The model under review builds one solid part; all positions refer to its coordinate system, in mm. A direction names the side the tool comes from. Round coordinates to 2 decimals unless told otherwise and drop trailing zeros. Order: outer loops, then holes, each group sorted by start corner. A loop starts at its lowest first (then second) coordinate and runs counter-clockwise, first axis right, second up.
1) Mouldability with a two-part tool opening along X and no side actions: class faces 4 (the face through (180.462, 10.81, -33.792)), 5 (the face through (239.15, -458.02, -15.02)), 6 (the face through (329.074, -455, -23)) as pulls with the +X half, pulls with the -X half, needs draft (parallel to the pull), parting line crosses it, or undercut.
2) Consider section A-A (z = 0). Give the boundary of the cut face in (x, y).
3) Consider section C-C (y = 411.5). Give the boundary of the cut face in (x, z).
4) Machinability: for faces 1 (the face through (-284, 306.407, -23)), 2 (the face through (-88.72, 495.28, -2.2)), 3 (the face through (-379.026, 381.199, -2.198)), which of the approach directions +Z, -Z, +X, -X, +Y, -Y give a long, thin tool a straight path to every point of the face, cutting with its end or side? Answer none if there is none.
5) To check wall thickness, follow L1, parallel to X at y = -121, z = 2.5; L2, parallel to X at y = -84.5, z = -23; L3, parallel to Y at x = 105, z = -45. State the ranges of each line that lie inside material, in increasing order.
6) Consider section B-B (x = 29.5). Give the boundary of the cut face in (y, z), then the cut area to 3 significant figures.
7) Clearance check with flat-ended pins moving along their axes: P1, Ø10, axis at x = -288.5, z = 9, coming from the +Y side; P2, Ø4, axis at y = -275, z = 21.5, coming from the +X side; P3, Ø2, axis at y = 147, z = 47.5, coming from the -X side. State where each tip first meets the part, or that it passes through.
8) Consider section D-D (y = -394.5). Give the boundary of the cut face in (x, z).
from build123d import *

# Parameters (mm, degrees)
SKETCH8_R   = 60
SKETCH8_R_2 = 50


with BuildPart() as part:
    # Sweep-Thin1: sweep along a path in Sketch1
    with BuildLine(Plane.XY) as sweep_thin1_path:
        Line((-329.073983606, 306.407118431), (-329.073983606, 445.327817433))
        Line((-329.073983606, 445.327817433), (143.609908522, 445.327817433))
        Line((143.609908522, 445.327817433), (143.609908522, -410.327817433))
        Line((143.609908522, -410.327817433), (329.073983606, -410.327817433))
    # Sketch8 → Sweep-Thin1 (sweep)
    with BuildSketch(Plane(origin=(0, 306.407118431, 0), x_dir=(1, 0, 0), z_dir=(0, 1, 0))):
        with Locations((-329.073983606, 0)):
            Circle(SKETCH8_R)
        with Locations((-329.073983606, 0)):
            Circle(SKETCH8_R_2, mode=Mode.SUBTRACT)
    sweep(path=sweep_thin1_path.line, transition=Transition.RIGHT)


solid = part.part
Answer below:
1. face 4: undercut
1. face 5: needs draft
1. face 6: pulls with the +X half
2. outline: (-389.07, 306.41) - (-379.07, 306.41) - (-379.07, 495.33) - (193.61, 495.33) - (193.61, -360.33) - (329.07, -360.33) - (329.07, -350.33) - (203.61, -350.33) - (203.61, 505.33) - (-389.07, 505.33) - close; (-279.07, 306.41) - (-269.07, 306.41) - (-269.07, 385.33) - (83.61, 385.33) - (83.61, -470.33) - (329.07, -470.33) - (329.07, -460.33) - (93.61, -460.33) - (93.61, 395.33) - (-279.07, 395.33) - close
3. outline: (-295.25, -49.55) - (109.78, -49.55) arc R60 ccw (long way) to (109.78, 49.55) - (-295.25, 49.55) arc R60 ccw (long way) to start; hole (-295.25, -36.82) - (109.78, -36.82) arc R50 ccw (long way) to (109.78, 36.82) - (-295.25, 36.82) arc R50 ccw (long way) to start
4. face 1: +Z, -Z, -X, -Y
4. face 2: none
4. face 3: -Y
5. L1: x = 83.66 to 93.67, 193.55 to 203.56
5. L2: x = 88.19 to 99.21, 188.01 to 199.03
5. L3: y = -450.01 to 423.53, 467.12 to 485.01
6. outline: circle Ø120 at (445.33, 0); hole circle Ø100 at (445.33, 0)
6. area: 3,460 mm2
7. P1: stops at y = 505.19
7. P2: stops at x = 200.35
7. P3: stops at x = 105.69
8. outline: (159.44, -57.87) - (329.07, -57.87) - (329.07, -47.43) - (159.44, -47.43) arc R50 cw (long way) to (159.44, 47.43) - (329.07, 47.43) - (329.07, 57.87) - (159.44, 57.87) arc R60 ccw (long way) to start
